Source: CAD feature listing. Evaluate the final solid. Frame: model axes, mm. A direction names the side the tool comes from. Coordinates: 2 decimals unless noted, no trailing zeros. Order: outer loops, then holes, each group sorted by start corner. A loop starts at its lowest first (then second) coordinate and runs counter-clockwise, first axis right, second up. Notation, with made-up numbers: (76.25, 20) - (113.25, 20) arc R19 cw to (113.25, 52) - close; hole circle Ø8 at (60, 6.5). An arc over 180 degrees is marked (long way). One line per question, with ' | ' between items. Start each with the question number.
(1) Draft query along Y for faces 1 (the flat face through (2, 40, 25)), 2 (the flat face through (0, 20, 25)), 3 (the flat face through (2, 0, 25)), 4 (the flat face through (15, 20, 32.08)). Return one class per face: +Y half, -Y half, draft (parallel to the pull), parting line (faces both ways), or undercut.
(2) Section D-D (z = 43.5). Return the cut outline in (x, y), then the cut area to 3 significant figures.
(3) Line query: line 1 along Y through (x, z) = (19.75, 12); line 2 along X through (y, z) = (24, 40); line 3 along Z through (x, y) = (14, 21.5). Output: solid intervals per line, ascending.
(4) Section B-B (x = 8.75). Return the cut outline in (y, z), then the cut area to 3 significant figures.
(5) Contact query for flat-ended pins moving along their axis: P1, Ø10, axis at x = 18.5, z = 27.5, coming from the -Y side; P2, Ø1.2, axis at x = 19, y = 27, coming from the -Z side; P3, Ø14.5, axis at x = 11, y = 18.5, coming from the +Z side; P4, Ø3, axis at x = 16.5, y = 20.5, coming from the -Z side. Output: stop coordinate, or through.
(6) Section A-A (y = 13). Return the cut outline in (x, z), then the cut area to 3 significant figures.
(7) Section C-C (z = 25.5). Return the cut outline in (x, y).
(8) Access query for faces 5 (the flat face through (15, 11, 21)), 6 (the flat face through (15, 27, 5)), 7 (the flat face through (15, 29, 20)), 8 (the flat face through (15, 15, 18)), 9 (the flat face through (15, 20, 36.08)). Directions: +Z, -Z, +X, -X, +Y, -Y. A direction counts if a zero-diameter tool reaches every point of the face in a straight line with its end or side. Return the directions, or none.
from build123d import *

# Parameters (mm, degrees)
F0_W     = 40
F0_H     = 50
F1_DEPTH = 5
F3_DEPTH = 20


with BuildPart() as f1:
    # F0 (on Right) → F1 (new body)
    with BuildSketch(Plane.YZ):
        with Locations((20, 25)):
            Rectangle(F0_W, F0_H)
    extrude(amount=F1_DEPTH)

    # F2 (on face) → F3 (join)
    with BuildSketch(Plane.YZ.offset(5)):
        Polygon((11, 36.08), (11, 5), (15, 5), (15, 32.08), (25, 32.08), (25, 5), (29, 5), (29, 36.08), align=None)
    extrude(amount=F3_DEPTH)


solid = f1.part
Response values:
1) face 1: +Y half | face 2: draft | face 3: -Y half | face 4: undercut
2) outline: (0, 0) - (5, 0) - (5, 40) - (0, 40) - close | area: 200 mm²
3) line 1: y = 11 to 15, 25 to 29 | line 2: x = 0 to 5 | line 3: z = 32.08 to 36.08
4) outline: (11, 5) - (15, 5) - (15, 32.08) - (25, 32.08) - (25, 5) - (29, 5) - (29, 36.08) - (11, 36.08) - close | area: 289 mm²
5) P1: stops at y = 11 | P2: stops at z = 5 | P3: stops at z = 50 | P4: stops at z = 32.08
6) outline: (0, 0) - (5, 0) - (5, 5) - (25, 5) - (25, 36.08) - (5, 36.08) - (5, 50) - (0, 50) - close | area: 872 mm²
7) outline: (0, 0) - (5, 0) - (5, 11) - (25, 11) - (25, 15) - (5, 15) - (5, 25) - (25, 25) - (25, 29) - (5, 29) - (5, 40) - (0, 40) - close
8) face 5: +Z, -Z, +X, -Y | face 6: -Z, +X, +Y, -Y | face 7: +Z, -Z, +X, +Y | face 8: -Z, +X | face 9: +Z, +X, +Y, -Y
